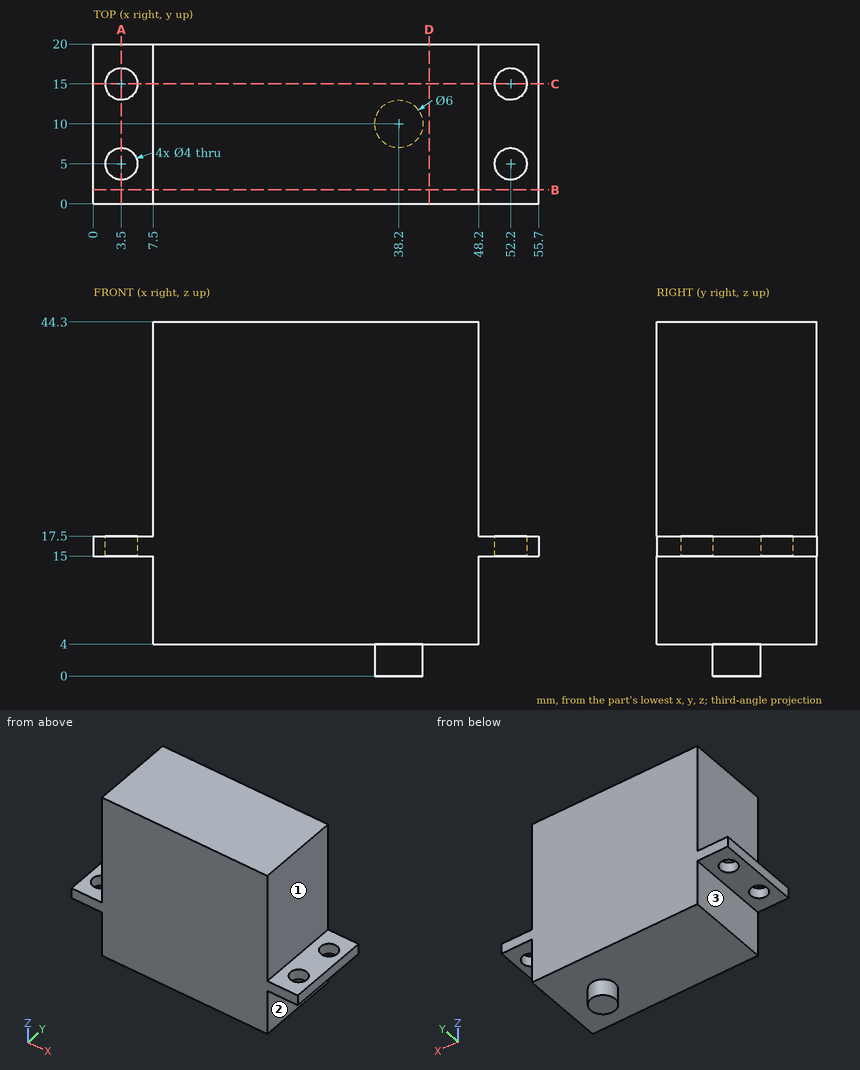
Verification items for this drawing (mm, ordinates from the low corner). A direction names the side the tool comes from. Give positions to 0.01 mm unless a question says otherwise; leave off trailing zeros. Write each loop counter-clockwise with the first axis right and the second up, starting at its lowest first coordinate (ties: lowest second). Pieces come first, ordered by that corner, then holes. Notation, with made-up numbers: (57.25, 31.25) - (80.25, 31.25) arc R21 ccw to (80.25, 46.25) - close; hole circle Ø5 at (10, 25). An arc over 180 degrees is marked (long way). Answer as CSV lines item,"result". Start each with the question number.
1. Sectioned sample at C-C (y = 15). Record the boundary of the cut face in (x, z), then the cut area to 3 significant figures.
2. Sectioned sample at A-A (x = 3.5). Record the boundary of the cut face in (y, z), then the cut area to 3 significant figures.
3. Thickness scan on line 1 (Y direction, x = 52, z = 16); line 2 (Z direction, x = 48, y = 1.75); line 3 (Z direction, x = 50, y = 2). Record the ranges inside material, lowest first.
4. Sectioned sample at B-B (y = 1.75). Record the boundary of the cut face in (x, z), then the cut area to 3 significant figures.
5. Set-up check for the marked faces 1, 2 and 3: record each of +Z, -Z, +X, -X, +Y, -Y from which the full face is reachable in a straight line by a thin tool's end or side.
6. Depth check by flat-ended pin: pin 1 (3 mm diameter, centred on x = 52.2, y = 5, fed in from +Z); pin 2 (4 mm diameter, centred on x = 50.5, y = 13.5, fed in from -Z); pin 3 (6 mm diameter, centred on x = 3.5, y = 13, fed in from +Z); pin 4 (10 mm diameter, centred on x = 23.5, y = 4, fed in from -Z). Enter the tip coordinate at first touch or a pass-through.
7. Sectioned sample at D-D (x = 42). Record the boundary of the cut face in (y, z), then the cut area to 3 significant figures.
Derived:
1,outline,"(0, 15) - (1.5, 15) - (1.5, 17.5) - (0, 17.5) - close; (5.5, 15) - (7.5, 15) - (7.5, 4) - (48.2, 4) - (48.2, 15) - (50.2, 15) - (50.2, 17.5) - (48.2, 17.5) - (48.2, 44.3) - (7.5, 44.3) - (7.5, 17.5) - (5.5, 17.5) - close; (54.2, 15) - (55.7, 15) - (55.7, 17.5) - (54.2, 17.5) - close"
1,area,"1,660 mm²"
2,outline,"(0, 15) - (3, 15) - (3, 17.5) - (0, 17.5) - close; (7, 15) - (13, 15) - (13, 17.5) - (7, 17.5) - close; (17, 15) - (20, 15) - (20, 17.5) - (17, 17.5) - close"
2,area,"30.0 mm²"
3,line 1,"0 to 3.01, 6.99 to 13.01, 16.99 to 20"
3,line 2,"4 to 44.3"
3,line 3,"15 to 17.5"
4,outline,"(0, 15) - (7.5, 15) - (7.5, 4) - (48.2, 4) - (48.2, 15) - (55.7, 15) - (55.7, 17.5) - (48.2, 17.5) - (48.2, 44.3) - (7.5, 44.3) - (7.5, 17.5) - (0, 17.5) - close"
4,area,"1,680 mm²"
5,face 1,"+Z, +X, +Y, -Y"
5,face 2,"-Z, +X, +Y, -Y"
5,face 3,"-Z, -X, +Y, -Y"
6,pin 1,"through"
6,pin 2,"z = 15"
6,pin 3,"z = 17.5"
6,pin 4,"z = 4"
7,outline,"(0, 4) - (20, 4) - (20, 44.3) - (0, 44.3) - close"
7,area,"806 mm²"
